Design review of the part built by this model. Coordinates are the model's own, in mm. A direction names the side the tool comes from. Round coordinates to 2 decimals unless told otherwise and drop trailing zeros. Write each loop counter-clockwise with the first axis right and the second up, starting at its lowest first coordinate (ties: lowest second). Pieces come first, ordered by that corner, then holes. Notation, with made-up numbers: (39.25, 9.25) - (93.25, 9.25) arc R16 cw to (93.25, 26.25) - close; hole circle Ø4 at (-10.75, 48.5). An arc over 180 degrees is marked (long way). Use one line per item in the form item = value.
Autodesk Inventor part; units mm, degrees
ref_plane "YZ Plane" through (0, 0, 0) normal (1, 0, 0) x (0, 1, 0)
ref_plane "XZ Plane" through (0, 0, 0) normal (0, 1, 0) x (-1, 0, 0)
ref_plane "XY Plane" through (0, 0, 0) normal (0, 0, 1) x (1, 0, 0)
sketch "Sketch1" plane through (0, 0, 0) normal (0, 0, 1) x (1, 0, 0)
  line L0 (15, -7) -> (-15, -7)
  line L1 (-15, -7) -> (-15, 7)
  line L2 (-15, 7) -> (15, 7)
  line L3 (15, 7) -> (15, -7)
  line L4 (15, -7) -> (-15, 7) construction
  line L5 (-15, -7) -> (15, 7) construction
  point P0 (0, 0)
  dimension "d0" = 30
  dimension "d1" = 14
extrude "Extrusion1" add sketch "Sketch1" along normal blind 35
sketch "Sketch3" plane through (15, -7, 0) normal (1, 0, 0) x (0, 0, -1)
  line L0 (0, 0) -> (-35, 0)
  line L1 (-17.5, 0) -> (-17.5, -2)
  arc A0 (-8.2129, 0) -> (-26.7871, 0) centre (-17.5, -2) ccw
  point P0 (0, 7)
  dimension "d4" = 2
  dimension "d5" = 19
extrude "Extrusion2" cut sketch "Sketch3" against normal blind 25
sketch "Sketch5" plane through (-15, 7, 0) normal (0, 1, 0) x (1, 0, 0)
  line L0 (30, 0) -> (0, 0)
  line L1 (30, -35) -> (0, -35)
  line L2 (0, -35) -> (0, -30.9)
  line L3 (0, 0) -> (0, -35)
  line L4 (0, -30.9) -> (2.75, -30.9)
  circle A0 centre (2.75, -30.9) radius 2
  line L5 (0, 0) -> (0, -4.1)
  line L6 (0, -4.1) -> (2.75, -4.1)
  circle A1 centre (2.75, -4.1) radius 2
  line L7 (2.75, -30.9) -> (10.75, -30.9)
  circle A2 centre (10.75, -30.9) radius 3.175
  point P0 (15, 0)
  dimension "d11" = 4.1
  dimension "d12" = 2.75
  dimension "d13" = 4
  dimension "d14" = 4.1
  dimension "d15" = 2.75
  dimension "d16" = 4
  dimension "d17" = 8
  dimension "d18" = 6.35
extrude "Extrusion3" cut sketch "Sketch5" against normal blind 100 contours A2
sketch "Sketch6" plane through (-15, 7, 0) normal (0, 1, 0) x (1, 0, 0)
  point P0 (15, 0)
sketch "Sketch7" plane through (15, -7, 0) normal (1, 0, 0) x (0, 0, -1)
  line L0 (0, 14) -> (-35, 14)
  line L1 (-35, 14) -> (-30, 14)
  line L2 (-30, 14) -> (-30, 9)
  line L3 (0, 14) -> (0, 0)
  line L4 (0, 14) -> (-5, 14)
  line L5 (-5, 14) -> (-5, 9)
  circle A0 centre (-30, 9) radius 3.175
  circle A1 centre (-5, 9) radius 3.175
  point P0 (0, 7)
  dimension "d21" = 5
  dimension "d22" = 5
  dimension "d23" = 5
  dimension "d24" = 5
  dimension "d25" = 6.35
  dimension "d26" = 6.35
extrude "Extrusion4" cut sketch "Sketch7" against normal blind 15
move or copy body "Move Body1" bodies to move or copy 1 copy no translate (-20, 0, 0)
move or copy body "Move Body2" bodies to move or copy 1 copy no translate (-5, 0, 0)
sketch "Sketch8" plane through (0, 0, 0) normal (1, 0, 0) x (0, 1, 0)
  point P0 (0, 0)
sketch "Sketch9" plane through (-40, 7, 0) normal (0, 1, 0) x (1, 0, 0)
  line L0 (30, -35) -> (0, -35)
  line L1 (0, -35) -> (0, -30.9)
  line L2 (0, 0) -> (0, -35)
  line L3 (0, -30.9) -> (3, -30.9)
  circle A0 centre (3, -30.9) radius 2
  line L4 (0, 0) -> (0, -4.1)
  line L5 (0, -4.1) -> (3, -4.1)
  circle A1 centre (3, -4.1) radius 2
  point P0 (40, 0)
  dimension "d35" = 4.1
  dimension "d36" = 3
  dimension "d37" = 4
  dimension "d38" = 4.1
  dimension "d39" = 4
  dimension "d40" = 3
extrude "Extrusion5" cut sketch "Sketch9" against normal blind 14
sketch "Sketch14" plane through (-40, 7, 35) normal (0, 0, 1) x (1, 0, 0)
  line L0 (30, 0) -> (0, 0)
  line L1 (30, 0) -> (25, 0)
  line L2 (25, 0) -> (25, -5)
  circle A0 centre (25, -5) radius 2
  point P0 (40, -7)
  dimension "d47" = 5
  dimension "d48" = 5
  dimension "d49" = 4
extrude "Extrusion6" cut sketch "Sketch14" against normal blind 3
sketch "Sketch15" plane through (-10, 7, 0) normal (0, 0, -1) x (-1, 0, 0)
  line L0 (0, -14) -> (0, 0)
  line L1 (0, 0) -> (5, 0)
  line L2 (0, 0) -> (30, 0)
  line L3 (5, 0) -> (5, -5)
  circle A0 centre (5, -5) radius 2
  point P0 (-10, -7)
  dimension "d52" = 5
  dimension "d53" = 5
  dimension "d54" = 4
extrude "Extrusion7" cut sketch "Sketch15" against normal blind 4
thread "Thread3"
thread "Thread4"
sketch "Sketch16" plane through (-40, -7, 0) normal (-1, 0, 0) x (0, 0, 1)
  line L0 (0, 14) -> (35, 14)
  line L1 (0, 14) -> (17.5, 14)
  line L2 (17.5, 14) -> (17.5, -2)
  circle A0 centre (17.5, -2) radius 7.5
  point P0 (0, 7)
  dimension "d61" = 16
  dimension "d62" = 15
extrude "Extrusion8" cut sketch "Sketch16" against normal blind 15
move or copy body "Move Body3" bodies to move or copy 1 copy no translate (25, 0, 0)
move or copy body "Move Body4" bodies to move or copy 1 copy no translate (10, 0, -15)
move or copy body "Move Body5" bodies to move or copy 1 copy no translate (-10, 0, 0)
sketch "Sketch17" plane through (15, -7, -15) normal (1, 0, 0) x (0, 0, -1)
  point P0 (-15, 7)
equation "\"d55\" = d54"
properties part number "Rb oven housing top-back" material "Copper"
Q1. Machinability: for faces 5 (the cylindrical face through (11.474, 3.352, -14.032)), 6 (the cylindrical face through (-4.94, 0.1, 19)), 7 (the cylindrical face through (2.68, 0.5, 2.32)), 8 (the cylindrical face through (7.6, 0.78, 12.07)), 9 (the cylindrical face through (8.526, 3.352, 19.032)), which of the approach directions +Z, -Z, +X, -X, +Y, -Y give a long, thin tool a straight path to every point of the face, cutting with its end or side? Answer none if there is none.
Calculated:
face_5 = -Z
face_6 = +Y, -Y
face_7 = +X, -Y
face_8 = +X
face_9 = +Z
Q2. We need section D-D on z = 15. Write out the cut boundary in (x, y) (3 decimals), then the cut area to 3 significant figures.
Calculated:
outline = (-15, -7) - (-13.786, -7) - (-13.786, 7) - (-15, 7) - close; (-10.214, -7) - (-7.295, -7) - (-7.295, 7) - (-10.214, 7) - close; (-1.205, -7) - (15, -7) - (15, -1.175) - (0, -1.175) - (0, 5.175) - (15, 5.175) - (15, 7) - (-1.205, 7) - close
area = 189 mm2
Q3. We need section B-B on y = 2. Write out the cut boundary in (x, z) (3 decimals), then the cut area to 3 significant figures.
Calculated:
outline = (-15, -15) - (8, -15) - (8, -13.175) - (0, -13.175) - (0, -6.825) - (15, -6.825) - (15, 11.825) - (0, 11.825) - (0, 18.175) - (8, 18.175) - (8, 20) - (-15, 20) - close; (12, -15) - (15, -15) - (15, -13.175) - (12, -13.175) - close; (12, 18.175) - (15, 18.175) - (15, 20) - (12, 20) - close; hole circle Ø4 at (-12, -10.9); hole circle Ø4 at (-12, 15.9); hole circle Ø6.35 at (-4.25, 15.9)
area = 788 mm2
Q4. Draft analysis for pull direction Y (two halves, no side actions). For faces 1 (the flat face through (0, -7, 16)), 2 (the flat face through (0, 7, 2)), 3 (the flat face through (0, 2, 15)), 4 (the flat face through (15, 2, 2)), state which applies: released by +Y, released by -Y, zero draft, split by the parting line, or undercut.
Calculated:
face_1 = released by -Y
face_2 = released by +Y
face_3 = undercut
face_4 = zero draft
Q5. We need section A-A on x = -12. Write out the cut boundary in (y, z), then the cut area to 3 significant figures.
Calculated:
outline = (-7, -15) - (7, -15) - (7, -12.9) - (-7, -12.9) - close; (-7, -8.9) - (7, -8.9) - (7, 13.9) - (-7, 13.9) - (-7, 9.73) arc R7.5 cw to (-7, -4.73) - close; (-7, 17.9) - (7, 17.9) - (7, 20) - (-7, 20) - close
area = 319 mm2
Q6. We need section C-C on x = 5. Write out the cut boundary in (y, z) (3 decimals), then the cut area to 3 significant figures.
Calculated:
outline = (-7, -15) - (7, -15) - (7, 20) - (-7, 20) - (-7, 11.787) arc R9.5 cw to (-7, -6.787) - close; hole circle Ø6.35 at (2, -10); hole circle Ø6.35 at (2, 15)
area = 323 mm2
Q7. To check wall thickness, follow line 1 along Z through (x, y) = (4.75, 2) (3 decimals); line 2 along X through (y, z) = (3, 15.9) (3 decimals); line 3 along X through (y, z) = (-1.5, 15.9) (3 decimals). State the ranges of each line that lie inside material, in increasing order. Write a range as from..to.
Calculated:
line_1 = -15..-13.175, -6.825..11.825, 18.175..20
line_2 = -15..-14, -10..-7.425, -1.075..0
line_3 = -15..-14, -10..-7.425, -1.075..15
Q8. For P1, Ø2.5, axis at x = 10, y = 2, coming from the -Z side; P2, Ø5, axis at x = -4.25, z = 15.9, coming from the -Y side; P3, Ø2.5, axis at x = 10, y = 2, coming from the +Z side; P4, Ø3, axis at x = 5, z = 7.5, coming from the -Y side, all flat-tipped, find the tip position at first contact; note any pin that passes through.
Calculated:
P1 = -7.08
P2 = through
P3 = 12.08
P4 = -2.07
